```python
from build123d import *
from build123d.topology import SkipClean

# Parameters (mm, degrees)
SALIENTE_EXTRUIR1_DEPTH      = 20
CORTAR_EXTRUIR1_START        = -3
CORTAR_EXTRUIR1_DEPTH        = 3
CORTAR_EXTRUIR2_DEPTH        = 3
SALIENTE_EXTRUIR4_START      = -20
SALIENTE_EXTRUIR4_DEPTH      = 20
CORTAR_EXTRUIR3_START        = -3
CORTAR_EXTRUIR3_DEPTH        = 3
CORTAR_EXTRUIR4_DEPTH        = 3
CROQUIS9_R                   = 2
CORTAR_EXTRUIR5_DEPTH        = 20
SALIENTE_EXTRUIR5_DEPTH      = 7
SALIENTE_EXTRUIR5_DEPTH_BACK = 27
CROQUIS11_R                  = 2
CORTAR_EXTRUIR6_DEPTH        = 10
REDONDEO1_R                  = 2
REDONDEO3_R                  = 2
CROQUIS12_W                  = 34
CROQUIS12_H                  = 34
CORTAR_EXTRUIR7_DEPTH        = 3


with BuildPart() as part:
    # Croquis1 → Saliente-Extruir1 (new body)
    with BuildSketch(Plane(origin=(0, 0, 0), x_dir=(1, 0, 0), z_dir=(0, 1, 0))):
        with BuildLine():
            Line((-44.472135955, 11.05572809), (-4.472135955, -8.94427191))
            ThreePointArc((-4.472135955, -8.94427191), (9.165086698, -4.000148225), (3.517298828, 9.361015381))
            Line((3.517298828, 9.361015381), (-34.952618119, 28.632724723))
            ThreePointArc((-34.952618119, 28.632724723), (-48.793203604, 24.762307253), (-44.472135955, 11.05572809))
        make_face()
    extrude(amount=SALIENTE_EXTRUIR1_DEPTH)

    # Croquis3 → Cortar-Extruir1 (cut)
    with BuildSketch(Plane(origin=(0, 20, 0), x_dir=(1, 0, 0), z_dir=(0, 1, 0)).offset(CORTAR_EXTRUIR1_START)):
        with BuildLine():
            Line((-34.952618119, 28.632724723), (-22.125927279, 22.20712578))
            Line((-22.125927279, 22.20712578), (-31.05572809, 4.347524158))
            Line((-31.05572809, 4.347524158), (-44.472135955, 11.05572809))
            ThreePointArc((-44.472135955, 11.05572809), (-31.206796396, 15.237692747), (-34.952618119, 28.632724723))
        make_face()
    extrude(amount=CORTAR_EXTRUIR1_DEPTH, mode=Mode.SUBTRACT)

    # Croquis5 → Cortar-Extruir2 (cut)
    with BuildSketch(Plane.XZ):
        with BuildLine():
            Line((-35.508565818, -28.934596744), (-22.125927279, -22.20712578))
            Line((-22.125927279, -22.20712578), (-31.05572809, -4.347524158))
            Line((-31.05572809, -4.347524158), (-44.472135955, -11.05572809))
            ThreePointArc((-44.472135955, -11.05572809), (-31.060560465, -15.518212321), (-35.508565818, -28.934596744))
        make_face()
    extrude(amount=-CORTAR_EXTRUIR2_DEPTH, mode=Mode.SUBTRACT)

    # Croquis6 → Saliente-Extruir4 (add)
    with BuildSketch(Plane(origin=(0, 20, 0), x_dir=(1, 0, 0), z_dir=(0, 1, 0)).offset(SALIENTE_EXTRUIR4_START)):
        with BuildLine():
            ThreePointArc((-50, 20), (-40, 30), (-30, 20))
            Line((-30, 20), (-30, 65))
            Line((-30, 65), (-50, 70))
            Line((-50, 70), (-50, 20))
        make_face()
    extrude(amount=SALIENTE_EXTRUIR4_DEPTH)

    # Croquis7 → Cortar-Extruir3 (cut)
    with BuildSketch(Plane(origin=(0, 20, 0), x_dir=(1, 0, 0), z_dir=(0, 1, 0)).offset(CORTAR_EXTRUIR3_START)):
        with BuildLine():
            Line((-50, 20), (-50, 35))
            Line((-50, 35), (-30, 35))
            Line((-30, 35), (-30, 20))
            ThreePointArc((-30, 20), (-40, 30), (-50, 20))
        make_face()
    extrude(amount=CORTAR_EXTRUIR3_DEPTH, mode=Mode.SUBTRACT)

    # Croquis8 → Cortar-Extruir4 (cut)
    with SkipClean():  # the faces are left unmerged after this step: merging them gives an invalid solid
        with BuildSketch(Plane.XZ):
            with BuildLine():
                Line((-30, -20), (-30, -35))
                Line((-30, -35), (-50, -35))
                Line((-50, -35), (-50, -20))
                ThreePointArc((-50, -20), (-40, -30), (-30, -20))
            make_face()
        extrude(amount=-CORTAR_EXTRUIR4_DEPTH, mode=Mode.SUBTRACT)

    # Croquis9 → Cortar-Extruir5 (cut)
    with SkipClean():  # the faces are left unmerged after this step: merging them gives an invalid solid
        with BuildSketch(Plane(origin=(-30, 0, 0), x_dir=(0, 0, -1), z_dir=(1, 0, 0))):
            with Locations((60, 10.062568572)):
                Circle(CROQUIS9_R)
            with Locations((50, 10.062568572)):
                Circle(CROQUIS9_R)
        extrude(amount=-CORTAR_EXTRUIR5_DEPTH, mode=Mode.SUBTRACT)

    # Croquis10 → Saliente-Extruir5 (add, two sides: drawn at the far end of the back side and taken through both)
    with SkipClean():  # the faces are left unmerged after this step: merging them gives an invalid solid
        with BuildSketch(Plane(origin=(0, 20, 0), x_dir=(1, 0, 0), z_dir=(0, 1, 0)).offset(-SALIENTE_EXTRUIR5_DEPTH_BACK)):
            with BuildLine():
                Line((0, -10), (17, -10))
                Line((17, -10), (17, 0))
                Line((17, 0), (10, 0))
                ThreePointArc((10, 0), (0, 10), (-10, 0))
                Line((-10, 0), (-17, 0))
                Line((-17, 0), (-17, -1.677390217))
                Line((-17, -1.677390217), (-17, -10))
                Line((-17, -10), (0, -10))
            make_face()
        extrude(amount=SALIENTE_EXTRUIR5_DEPTH + SALIENTE_EXTRUIR5_DEPTH_BACK)

    # Croquis11 → Cortar-Extruir6 (cut)
    with SkipClean():  # the faces are left unmerged after this step: merging them gives an invalid solid
        with BuildSketch(Plane(origin=(0, 0, 0), x_dir=(-1, 0, 0), z_dir=(0, 0, -1))):
            with Locations((13.5, 23.5)):
                Circle(CROQUIS11_R)
            with Locations((-13.5, 23.5)):
                Circle(CROQUIS11_R)
            with Locations((-13.5, -3.5)):
                Circle(CROQUIS11_R)
            with Locations((13.5, -3.5)):
                Circle(CROQUIS11_R)
        extrude(amount=-CORTAR_EXTRUIR6_DEPTH, mode=Mode.SUBTRACT)

    # Redondeo1
    redondeo1_edges = [part.edges().sort_by_distance(p)[0] for p in [
        (-26.590827684, 20, -13.277324969),
        (-26.590827684, 0, -13.277324969),
        (-40, 20, -35),
        (-40, 0, -35),
    ]]
    fillet(redondeo1_edges, radius=REDONDEO1_R)

    # Redondeo3
    redondeo3_edges = [part.edges().sort_by_distance(p)[0] for p in [
        (-40, 0, -67.5),
        (-40, 20, -67.5),
    ]]
    fillet(redondeo3_edges, radius=REDONDEO3_R)

    # Croquis12 → Cortar-Extruir7 (cut)
    with SkipClean():  # the faces are left unmerged after this step: merging them gives an invalid solid
        with BuildSketch(Plane.XY.offset(10)):
            with Locations((0, 10)):
                Rectangle(CROQUIS12_W, CROQUIS12_H)
        extrude(amount=-CORTAR_EXTRUIR7_DEPTH, mode=Mode.SUBTRACT)


solid = part.part
```
Design review of the part built by this model. Coordinates are the model's own, in mm. A direction names the side the tool comes from. Coordinates: 2 decimals unless noted, no trailing zeros. Order: outer loops, then holes, each group sorted by start corner. A loop starts at its lowest first (then second) coordinate and runs counter-clockwise, first axis right, second up. Notation, with made-up numbers: (22.25, 11) -> (71.25, 11) arc R32 cw to (71.25, 39) -> close; hole circle Ø9 at (10, 10). An arc over 180 degrees is marked (long way). One line per item, written item: value. Start each with the question number.
Q1. Tool access review of faces 1 (the flat face through (-11.9, -2, 0)), 2 (the cylindrical face through (-40.14, 0.57, -35.6)), 3 (the flat face through (14, 10, 0)), 4 (the flat face through (-11.9, 25, 0)), 5 (the flat face through (-30, 3, -24)): name each direction out of +Z, -Z, +X, -X, +Y, -Y from which nothing blocks a thin tool from reaching the whole face with its end or side.
Q2. Take a section at B-B, the plane y = 23.5. State the section outline as (x, z) points.
Q3. Insertion check: pin 1 Ø6 at (x, y) = (-38, 1.5) entering from +Z; pin 2 Ø3.5 at (y, z) = (10.06, -60) entering from -X; pin 3 Ø10 at (x, z) = (-40.5, -49.5) entering from +Y; pin 4 Ø7.5 at (y, z) = (6, 4) entering from -X. Each pin has a flat end and moves straight along its axis. Give the tip position at first contact, or say it passes through.
Q4. Take a section at D-D, the plane x = -5. State the section outline as (y, z) points.
Q5. Take a section at C-C, the plane z = -33. State the section outline as (x, y) points.
Q6. For probe 1 along Y at (x, z) = (-13.5, 4); probe 2 along Y at (x, z) = (-38, -50); probe 3 along X at (y, z) = (7, -48), list the stretches that pass through material, from the lowest coordinate up.
Q7. Take a section at A-A, the plane x = 13.5. State the section outline as (y, z) points, then the cut area to 3 significant figures.
Q8. Mouldability with a two-part tool opening along X and no side actions: class faces 6 (the flat face through (-13.01, 9.86, -17.64)), 7 (the flat face through (-26.53, 2.49, -13.4)), 8 (the cylindrical face through (-11.9, 22.3, 3.5)), 9 (the flat face through (0, 27, 0)) as pulls with the +X half, pulls with the -X half, needs draft (parallel to the pull), parting line crosses it, or undercut.
Values follow:
1. face 1: -Z, -X, -Y
1. face 2: +X, -X, -Y
1. face 3: -Z, +X, +Y, -Y
1. face 4: -Z, -X, +Y
1. face 5: -Y
2. outline: (-17, 0) -> (-15.5, 0) -> (-15.5, 7) -> (-17, 7) -> close; (-11.5, 0) -> (-10, 0) arc R10 ccw to (10, 0) -> (11.5, 0) -> (11.5, 7) -> (-11.5, 7) -> close; (15.5, 0) -> (17, 0) -> (17, 7) -> (15.5, 7) -> close
3. pin 1: stops at z = -6.52
3. pin 2: passes through
3. pin 3: stops at y = 20
3. pin 4: stops at x = -21.86
4. outline: (-7, -8.66) -> (0, -8.66) -> (0, -13.63) -> (20, -13.63) -> (20, -8.66) -> (27, -8.66) -> (27, 7) -> (-7, 7) -> close
5. outline: (-50, 3) -> (-30, 3) -> (-30, 17) -> (-50, 17) -> close
6. probe 1: y = -7 to -5.5, -1.5 to 21.5, 25.5 to 27
6. probe 2: y = 0 to 8.06, 12.06 to 20
6. probe 3: x = -50 to -30
7. outline: (-7, 0) -> (-5.5, 0) -> (-5.5, 7) -> (-7, 7) -> close; (-1.5, 0) -> (21.5, 0) -> (21.5, 7) -> (-1.5, 7) -> close; (25.5, 0) -> (27, 0) -> (27, 7) -> (25.5, 7) -> close
7. area: 182 mm2
8. face 6: pulls with the +X half
8. face 7: undercut
8. face 8: undercut
8. face 9: needs draft
